The model under review builds one solid part; all positions refer to its coordinate system, in mm. Face numbers are marked on the shaded views. A direction names the side the tool comes from. Give positions to 0.01 mm unless a question says otherwise; leave off trailing zeros. Order: outer loops, then holes, each group sorted by start corner. A loop starts at its lowest first (then second) coordinate and runs counter-clockwise, first axis right, second up. Notation, with made-up numbers: (78, -15.5) -> (84, -15.5) arc R9 cw to (84, -0.5) -> close; hole circle Ø8 at (71, -27). An arc over 180 degrees is marked (long way). Use one line per item in the form item = value.
```python
from build123d import *

# Parameters (mm, degrees)
SKETCH_2_W          = 60
SKETCH_2_H          = 70
EXTRUDE_1_DEPTH     = 15
SKETCH_7_W          = 55.5
SKETCH_7_H          = 9
CUT_EXTRUDE_3_DEPTH = 91.530456977
EXTRUDE_3_DEPTH     = 60


with BuildPart() as part:
    # 草图2 → 凸台-拉伸1 (new body)
    with BuildSketch(Plane(origin=(0, 0, 0), x_dir=(1, 0, 0), z_dir=(0, 1, 0))):
        with Locations((-4.452764977, 31.111751152)):
            Rectangle(SKETCH_2_W, SKETCH_2_H)
    extrude(amount=EXTRUDE_1_DEPTH)

    # 草图7 → 切除-拉伸3 (cut, through all)
    with BuildSketch(Plane.ZY.offset(34.452764977)):
        with Locations((-31.111751152, 10.5)):
            Rectangle(SKETCH_7_W, SKETCH_7_H)
    extrude(amount=-CUT_EXTRUDE_3_DEPTH, mode=Mode.SUBTRACT)

    # 草图8 → 凸台-拉伸3 (add)
    with BuildSketch(Plane.ZY.offset(34.452764977)):
        Polygon((-46.111751152, 0), (-16.111751152, 0), (-23.076751152, -12.144495667), (-25.861751152, -12.144495667), (-25.861751152, -2.537373778), (-36.361751152, -2.537373778), (-36.361751152, -12.144495667), (-39.146751152, -12.144495667), align=None)
    extrude(amount=-EXTRUDE_3_DEPTH)


solid = part.part
```
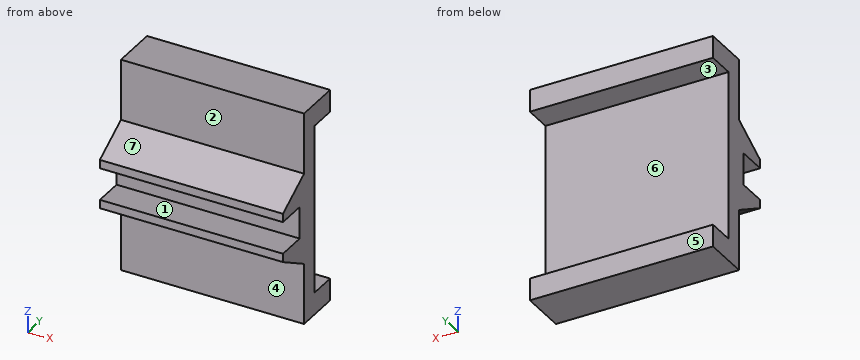
1. For L1, parallel to Z at x = -30, y = 12.75; L2, parallel to Y at x = 5.5, z = -4; L3, parallel to Z at x = 6, y = -3.5, list the stretches that pass through material, from the lowest coordinate up.
Values:
L1 = -66.11 to -58.86, -3.36 to 3.89
L2 = 0 to 6
L3 = -44.1 to -36.36, -25.86 to -18.12
2. Tool access review of the marked faces 1, 2, 3 and 4: name each direction out of +Z, -Z, +X, -X, +Y, -Y from which nothing blocks a thin tool from reaching the whole face with its end or side.
Values:
face_1 = +X, -X, -Y
face_2 = +Z, +X, -X, -Y
face_3 = +X, -X, +Y
face_4 = -Z, +X, -X, -Y
3. Add section D-D on z = -5. Give the boundary of the cut face in (x, y), then the cut area to 3 significant figures.
Values:
outline = (-34.45, 0) -> (25.55, 0) -> (25.55, 6) -> (-34.45, 6) -> close
area = 360 mm^2
4. The part is to be moulded in two halves that separate along Z. For the marked faces 5, 6 and 7, say which applies: +Z half, -Z half, draft (parallel to the pull), parting line (faces both ways), or undercut.
Values:
face_5 = draft
face_6 = undercut
face_7 = +Z half
5. Add section B-B on x = -18. Give the boundary of the cut face in (y, z).
Values:
outline = (-12.14, -39.15) -> (0, -46.11) -> (0, -66.11) -> (15, -66.11) -> (15, -58.86) -> (6, -58.86) -> (6, -3.36) -> (15, -3.36) -> (15, 3.89) -> (0, 3.89) -> (0, -16.11) -> (-12.14, -23.08) -> (-12.14, -25.86) -> (-2.54, -25.86) -> (-2.54, -36.36) -> (-12.14, -36.36) -> close
6. Add section A-A on y = 12.75. Give the boundary of the cut face in (x, z).
Values:
outline = (-34.45, -66.11) -> (25.55, -66.11) -> (25.55, -58.86) -> (-34.45, -58.86) -> close; (-34.45, -3.36) -> (25.55, -3.36) -> (25.55, 3.89) -> (-34.45, 3.89) -> close
7. For pin 1 Ø11.5 at (x, z) = (-7, -33.5) entering from -Y; pin 2 Ø10 at (x, z) = (-9, -51.5) entering from -Y; pin 3 Ø6 at (x, z) = (4, -47.5) entering from +Y; pin 4 Ø3 at (x, y) = (-5, -8) entering from +Z, all flat-tipped, find the tip position at first contact; note any pin that passes through.
Values:
pin_1 = -12.14
pin_2 = 0
pin_3 = 6
pin_4 = -19.84
8. Add section C-C on y = -9. Give the boundary of the cut face in (x, z), then the cut area to 3 significant figures.
Values:
outline = (-34.45, -40.95) -> (25.55, -40.95) -> (25.55, -36.36) -> (-34.45, -36.36) -> close; (-34.45, -25.86) -> (25.55, -25.86) -> (25.55, -21.27) -> (-34.45, -21.27) -> close
area = 551 mm^2
